The figure shows three views and two pictorial views of one solid part (mm, origin at its lowest corner). Answer the questions. A direction names the side the tool comes from. Round coordinates to 2 decimals unless told otherwise and drop trailing zeros. Loops run counter-clockwise (first coordinate to the right, second up) from the corner with the lowest first, then second, coordinate; pieces in that order, holes last. Notation, with made-up numbers: (71.25, -33) -> (80.25, -33) arc R26 ccw to (80.25, -9) -> close; hole circle Ø6 at (57, 60.25). An arc over 180 degrees is marked (long way). Put each result on its own line as item: value.
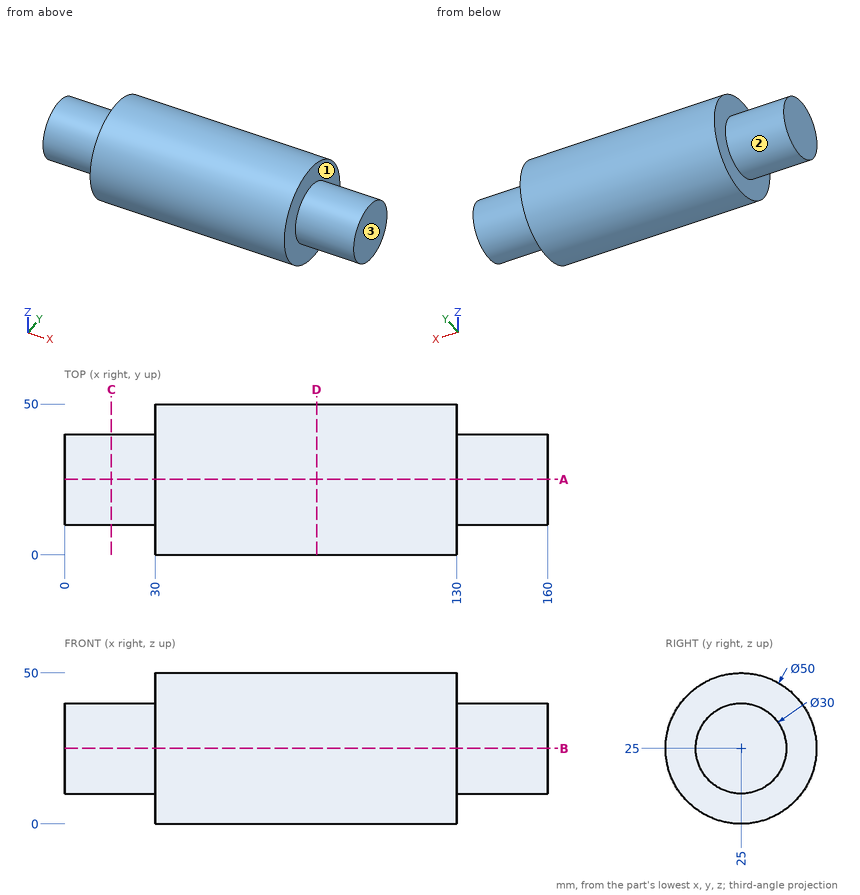
Item 1: Which of the six approach directions +Z, -Z, +X, -X, +Y, -Y give full straight-line access (tool end or side, diameter ignored) to the marked faces 1, 2 and 3?
Derived:
face 1: +X
face 2: -X
face 3: +Z, -Z, +X, +Y, -Y
Item 2: The part is cut by section C-C (x = 15.5). Determine the outline of the cut face in (y, z).
Derived:
outline: circle Ø30 at (25, 25)
Item 3: Flat-ended cylindrical pins translate along their axes: pin 1 Ø2 at (x, y) = (99, 27.5) entering from +Z; pin 2 Ø1 at (y, z) = (33, 42) entering from -X; pin 3 Ø5 at (y, z) = (43, 25.5) entering from +X. Find the tip coordinate at first contact, or state that the pin passes through.
Derived:
pin 1: stops at z = 49.95
pin 2: stops at x = 30
pin 3: stops at x = 130
Item 4: The part is cut by section A-A (y = 25). Determine the outline of the cut face in (x, z).
Derived:
outline: (0, 10) -> (30, 10) -> (30, 0) -> (130, 0) -> (130, 10) -> (160, 10) -> (160, 40) -> (130, 40) -> (130, 50) -> (30, 50) -> (30, 40) -> (0, 40) -> close
Item 5: The part is cut by section D-D (x = 83.5). Determine the outline of the cut face in (y, z), then the cut area to 3 significant figures.
Derived:
outline: circle Ø50 at (25, 25)
area: 1,960 mm^2
Item 6: Find the intervals of material crossed by line 1 along X through (y, z) = (31.5, 9); line 2 along Z through (x, y) = (19.5, 24.5); line 3 along Y through (x, z) = (72.5, 25), in increasing order.
Derived:
line 1: x = 30 to 130
line 2: z = 10.01 to 39.99
line 3: y = 0 to 50
